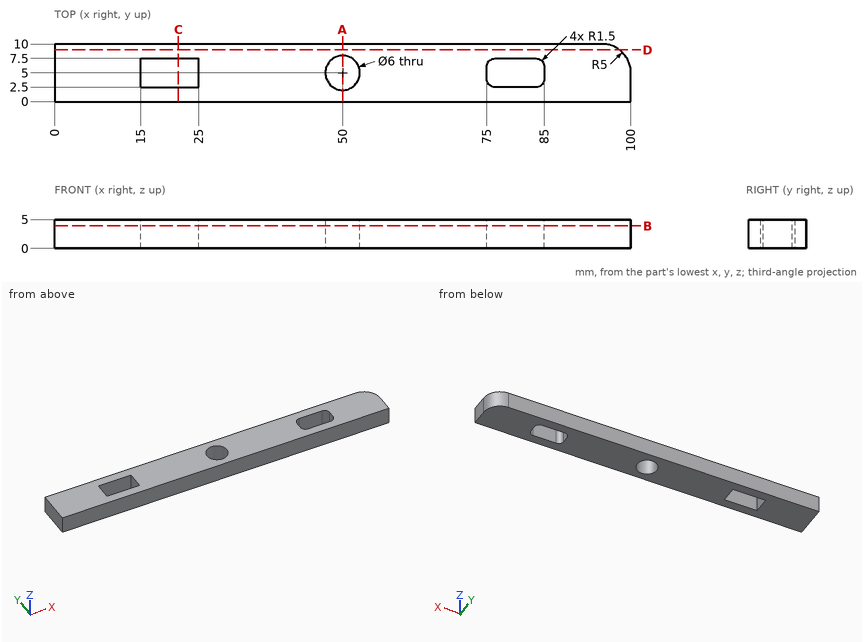
Geometry check sheet. Reference: drawing and pictorial views, mm from the part's lowest x, y, z. Give positions to 0.01 mm unless a question says otherwise; leave off trailing zeros. Order: outer loops, then holes, each group sorted by start corner. A loop starts at its lowest first (then second) coordinate and runs counter-clockwise, first axis right, second up. Notation, with made-up numbers: M -34,41.5 L 25,41.5 A17 cw 25,47.5 Z; hole C 85.25,76 d7. An arc over 180 degrees is marked long. Answer as a JSON object with one key per item and string values. Group by question number.
1) Cross-section at D-D (y = 9). Enter the section's corners in (x, z).
2) Cross-section at C-C (x = 21.5). Enter the section's corners in (y, z).
3) Cross-section at A-A (x = 50). Enter the section's corners in (y, z), then the cut area to 3 significant figures.
4) Cross-section at B-B (z = 3.9). Enter the section's corners in (x, y), then the cut area to 3 significant figures.
5) Scan lines: line 1 along Y through (x, z) = (50, 3.8); line 2 along Y through (x, z) = (16, 2.25); line 3 along X through (y, z) = (8.25, 3.4). Record each from-to range of solid material in increasing order. Write a range as [from, to].
6) Depth check by flat-ended pin: pin 1 Ø2 at (y, z) = (7.5, 2.5) entering from +X; pin 2 Ø1.5 at (x, z) = (19.5, 3) entering from -Y. Enter the tip coordinate at first touch or a pass-through.
Result sheet:
{
 "1": {"outline": "M 0,0 L 98,0 L 98,5 L 0,5 Z"},
 "2": {"outline": "M 0,0 L 2.5,0 L 2.5,5 L 0,5 Z; M 7.5,0 L 10,0 L 10,5 L 7.5,5 Z"},
 "3": {"outline": "M 0,0 L 2,0 L 2,5 L 0,5 Z; M 8,0 L 10,0 L 10,5 L 8,5 Z", "area": "20.0 mm2"},
 "4": {"outline": "M 0,0 L 100,0 L 100,5 A5 ccw 95,10 L 0,10 Z; hole M 15,2.5 L 25,2.5 L 25,7.5 L 15,7.5 Z; hole C 50,5 d6; hole M 75,4 A1.5 ccw 76.5,2.5 L 83.5,2.5 A1.5 ccw 85,4 L 85,6 A1.5 ccw 83.5,7.5 L 76.5,7.5 A1.5 ccw 75,6 Z", "area": "868 mm2"},
 "5": {"line 1": "y = [0, 2], [8, 10]", "line 2": "y = [0, 2.5], [7.5, 10]", "line 3": "x = [0, 98.8]"},
 "6": {"pin 1": "stops at x = 99.77", "pin 2": "stops at y = 0"}
}
